```python
from build123d import *

# Parameters (mm, degrees)
SKETCH_1_R          = 14.5
SKETCH_1_R_2        = 12.5
EXTRUDE_1_DEPTH     = 15
EXTRUDE_START       = 10
SKETCH_1_3_W        = 150
SKETCH_1_3_H        = 150
SKETCH_1_3_R        = 12.5
EXTRUDE_1_2_DEPTH   = 10
SKETCH_2_R          = 2.5
CUT_EXTRUDE_1_DEPTH = 10


with BuildPart() as part:
    # 草图1 → Extrude 1 (new body)
    with BuildSketch(Plane.XY):
        Circle(SKETCH_1_R)
        Circle(SKETCH_1_R_2, mode=Mode.SUBTRACT)
    extrude(amount=-EXTRUDE_1_DEPTH)

    # 草图1<3> → Extrude 1 2 (add)
    with BuildSketch(Plane.XY.offset(EXTRUDE_START)):
        Rectangle(SKETCH_1_3_W, SKETCH_1_3_H)
        Circle(SKETCH_1_3_R, mode=Mode.SUBTRACT)
    extrude(amount=-EXTRUDE_1_2_DEPTH)

    # 草图2 → 切除-拉伸1 (cut)
    with BuildSketch(Plane.XY.offset(10)):
        with Locations((-60, 60)):
            Circle(SKETCH_2_R)
        with Locations((0, 60)):
            Circle(SKETCH_2_R)
        with Locations((60, 60)):
            Circle(SKETCH_2_R)
        with Locations((60, -60)):
            Circle(SKETCH_2_R)
        with Locations((0, -60)):
            Circle(SKETCH_2_R)
        with Locations((-60, -60)):
            Circle(SKETCH_2_R)
    extrude(amount=-CUT_EXTRUDE_1_DEPTH, mode=Mode.SUBTRACT)


solid = part.part
```
Source: CAD feature listing. Evaluate the final solid. Frame: model axes, mm. Coordinates: 2 decimals unless noted, no trailing zeros. Loops run counter-clockwise (first coordinate to the right, second up) from the corner with the lowest first, then second, coordinate; pieces in that order, holes last. Notation, with made-up numbers: M 29.25,58.25 L 81.25,58.25 A30 cw 81.25,97.25 Z; hole C 29,20 d3. An arc over 180 degrees is marked long. Put each result on its own line as item: value. Start each with the question number.
1) Cut plane C-C on y = -60. Return the cut outline in (x, z), then the cut area to 3 significant figures.
2) Cut plane A-A on x = 0. Return the cut outline in (y, z).
3) Cut plane B-B on z = 2.75. Return the cut outline in (x, y).
4) Contact query for flat-ended pins moving along their axis: pin 1 Ø6 at (x, y) = (27, -16.5) entering from -Z; pin 2 Ø5 at (y, z) = (-55, -4.5) entering from +X (1 decimal). Output: stop coordinate, or through.
5) Pull-direction query (Y, two-part tool) for faces 1 (the face through (6.691, -12.864, -7.395)), 2 (the face through (-1, 18, 0)), 3 (the face through (-0.54, 57.56, 5.07)); classes: pulls with the +Y half, pulls with the -Y half, needs draft (parallel to the pull), parting line crosses it, or undercut.
6) Ray query, L1, parallel to Y at x = 0, z = 7.5; L2, parallel to Y at x = 60, z = 6.25; L3, parallel to Y at x = -0.5, z = 4.5. Return the intervals inside material, ascending. Write a range as from..to.
7) Cut plane D-D on x = -60. Return the cut outline in (y, z), then the cut area to 3 significant figures.
The answers:
1. outline: M -75,0 L -62.5,0 L -62.5,10 L -75,10 Z; M -57.5,0 L -2.5,0 L -2.5,10 L -57.5,10 Z; M 2.5,0 L 57.5,0 L 57.5,10 L 2.5,10 Z; M 62.5,0 L 75,0 L 75,10 L 62.5,10 Z
1. area: 1,350 mm²
2. outline: M -75,0 L -62.5,0 L -62.5,10 L -75,10 Z; M -57.5,0 L -14.5,0 L -14.5,-15 L -12.5,-15 L -12.5,10 L -57.5,10 Z; M 12.5,-15 L 14.5,-15 L 14.5,0 L 57.5,0 L 57.5,10 L 12.5,10 Z; M 62.5,0 L 75,0 L 75,10 L 62.5,10 Z
3. outline: M -75,-75 L 75,-75 L 75,75 L -75,75 Z; hole C -60,-60 d5; hole C -60,60 d5; hole C 0,0 d25; hole C 0,-60 d5; hole C 0,60 d5; hole C 60,-60 d5; hole C 60,60 d5
4. pin 1: stops at z = 0
4. pin 2: passes through
5. face 1: parting line crosses it
5. face 2: needs draft
5. face 3: undercut
6. L1: y = -75..-62.5, -57.5..-12.5, 12.5..57.5, 62.5..75
6. L2: y = -75..-62.5, -57.5..57.5, 62.5..75
6. L3: y = -75..-62.45, -57.55..-12.49, 12.49..57.55, 62.45..75
7. outline: M -75,0 L -62.5,0 L -62.5,10 L -75,10 Z; M -57.5,0 L 57.5,0 L 57.5,10 L -57.5,10 Z; M 62.5,0 L 75,0 L 75,10 L 62.5,10 Z
7. area: 1,400 mm²
